Could you check a few things on this model? Use its own coordinates, in mm. Face numbers are marked on the shaded views. A direction names the side the tool comes from. Round coordinates to 2 decimals unless told otherwise and drop trailing zeros. Loops run counter-clockwise (first coordinate to the right, second up) from the corner with the lowest first, then second, coordinate; pieces in that order, holes last. Notation, with made-up numbers: (17.5, 63.25) -> (60.5, 63.25) arc R14 cw to (60.5, 83.25) -> close; hole circle Ø10 at (10, -35.75). An arc over 180 degrees is marked (long way). Put each result on its own line as item: value. Start each with the question number.
1. Imagine slicing it at A-A, the plane x = 0. Please give me the cut outline in (y, z), and give its area (3 significant figures).
2. Which directions (+Z, -Z, +X, -X, +Y, -Y) give clear straight access to the entire face, cutting with the end or side of a thin tool? Please do the marked faces 1, 2 and 3.
3. Imagine slicing it at B-B, the plane y = 8. Please give me the cut outline in (x, z).
4. I'm going to push flat-ended pins straight in: P1, Ø7, axis at x = 16, y = 12, coming from the +Z side; P2, Ø5, axis at y = 12, z = 8.5, coming from the +X side; P3, Ø1.2, axis at y = 10.5, z = 8.5, coming from the +X side. Where does each tip first touch, or does it pass through?
5. Imagine slicing it at D-D, the plane x = 14. Please give me the cut outline in (y, z).
6. If we mould it in two halves opening along Z, with no side actions, what happens to the marked faces 4, 5 and 6? For each: pulls with the +Z half, pulls with the -Z half, needs draft (parallel to the pull), parting line crosses it, or undercut.
7. I need wall thicknesses on line 1 (X direction, y = 2.65, z = -8); line 2 (X direction, y = 7.5, z = 10); line 3 (Y direction, x = 2.5, z = -10.75). Which ranges of each line are inside material? Lowest first, please. Write a range as [from, to].
8. Imagine slicing it at C-C, the plane y = 4.5. Please give me the cut outline in (x, z).
```python
from build123d import *

# Parameters (mm, degrees)
SKETCH1_R           = 1.05
BOSS_EXTRUDE1_DEPTH = 6
SKETCH2_W           = 14
SKETCH2_H           = 25
SKETCH2_W_2         = 6
SKETCH2_H_2         = 22
BOSS_EXTRUDE2_DEPTH = 10
FILLET1_R           = 1
CUT_EXTRUDE2_START  = -6
CUT_EXTRUDE2_DEPTH  = 6
FILLET2_R           = 2
CUT_EXTRUDE3_DEPTH  = 2
CUT_EXTRUDE4_REACH  = 36.587
SKETCH9_R           = 1
BOSS_EXTRUDE3_DEPTH = 1
FILLET3_R           = 1
SKETCH13_R          = 2
CUT_EXTRUDE5_DEPTH  = 2
CUT_EXTRUDE6_DEPTH  = 10
SKETCH15_R          = 1
CUT_EXTRUDE7_DEPTH  = 32.436443819
FILLET4_R           = 5


with BuildPart() as part:
    # Sketch1 → Boss-Extrude1 (new body)
    with BuildSketch(Plane(origin=(0, 0, 0), x_dir=(1, 0, 0), z_dir=(0, 1, 0))):
        Polygon((19, -4.5), (19, 5), (19, 12.5), (-19, 12.5), (-19, 5), (-19, -4.5), (-19, -5), (-19, -12.5), (19, -12.5), (19, -5), align=None)
        with Locations(Location((16, -8, 0), (0, 0, 270))):
            Circle(SKETCH1_R, mode=Mode.SUBTRACT)
        with Locations(Location((0, -8, 0), (0, 0, 270))):
            Circle(SKETCH1_R, mode=Mode.SUBTRACT)
        with Locations(Location((16, 8, 0), (0, 0, 270))):
            Circle(SKETCH1_R, mode=Mode.SUBTRACT)
        with Locations(Location((0, 8, 0), (0, 0, 270))):
            Circle(SKETCH1_R, mode=Mode.SUBTRACT)
        with Locations(Location((-16, -8, 0), (0, 0, 270))):
            Circle(SKETCH1_R, mode=Mode.SUBTRACT)
        with Locations(Location((-16, 8, 0), (0, 0, 270))):
            Circle(SKETCH1_R, mode=Mode.SUBTRACT)
    extrude(amount=BOSS_EXTRUDE1_DEPTH)

    # Sketch2 → Boss-Extrude2 (add)
    with BuildSketch(Plane(origin=(0, 6, 0), x_dir=(1, 0, 0), z_dir=(0, 1, 0))):
        with Locations((-12, 0)):
            Rectangle(SKETCH2_W, SKETCH2_H)
        with Locations((8, 0)):
            Rectangle(SKETCH2_W_2, SKETCH2_H_2)
    extrude(amount=BOSS_EXTRUDE2_DEPTH)

    # Fillet1
    fillet1_edges = [part.edges().sort_by_distance(p)[0] for p in [
        (8, 6, -11),
        (8, 6, 11),
    ]]
    fillet(fillet1_edges, radius=FILLET1_R)

    # Sketch7 → Cut-Extrude2 (cut)
    with BuildSketch(Plane(origin=(11, 0, 0), x_dir=(0, 0, -1), z_dir=(1, 0, 0)).offset(CUT_EXTRUDE2_START)):
        Polygon((-11, 11), (-9, 16), (9, 16), (11, 11), (15.487403983, 11), (15.487403983, 19.998448993), (-12.222391387, 19.998448993), (-12.222391387, 11), align=None)
    extrude(amount=CUT_EXTRUDE2_DEPTH, mode=Mode.SUBTRACT)

    # Fillet2
    fillet2_edges = [part.edges().sort_by_distance(p)[0] for p in [
        (8, 11, 11),
        (8, 16, 9),
        (8, 16, -9),
        (8, 11, -11),
    ]]
    fillet(fillet2_edges, radius=FILLET2_R)

    # Sketch8 → Cut-Extrude3 (cut)
    with BuildSketch(Plane(origin=(11, 0, 0), x_dir=(0, 0, -1), z_dir=(1, 0, 0))):
        Polygon((-5.690598923, 11), (-6.845299462, 13), (-9.154700538, 13), (-10.309401077, 11), (-9.154700538, 9), (-6.845299462, 9), align=None)
    cut_extrude3 = extrude(amount=-CUT_EXTRUDE3_DEPTH, mode=Mode.SUBTRACT)

    # Sketch9 → Cut-Extrude4 (cut, up to next)
    with BuildSketch(Plane(origin=(9, 0, 0), x_dir=(0, 0, -1), z_dir=(1, 0, 0)), mode=Mode.PRIVATE) as cut_extrude4_sk1:
        with Locations((-8, 11)):
            Circle(SKETCH9_R)
    cut_extrude4_tool1 = extrude(cut_extrude4_sk1.sketch, amount=-CUT_EXTRUDE4_REACH, mode=Mode.PRIVATE) & part.part
    cut_extrude4 = cut_extrude4_tool1.solids().sort_by_distance((9, 11, 8))[0]
    add(cut_extrude4, mode=Mode.SUBTRACT)

    # Mirror1: Cut-Extrude3, Cut-Extrude4 across plane
    add(cut_extrude3.mirror(Plane.XY), mode=Mode.SUBTRACT)
    add(cut_extrude4.mirror(Plane.XY), mode=Mode.SUBTRACT)

    # Sketch11 → Boss-Extrude3 (add, symmetric)
    with BuildSketch(Plane.XY):
        Polygon((19, 6), (11, 16), (11, 6), align=None)
    extrude(amount=BOSS_EXTRUDE3_DEPTH, both=True)

    # Fillet3
    # the kernel refuses this fillet: 1 mm, written as the material it adds along each edge
    with BuildSketch(Plane(origin=(8.5, 6, 1), x_dir=(0, 1, 0), z_dir=(1, 0, 0))) as fillet3_piece_1_section:
        with BuildLine():
            CenterArc((FILLET3_R, FILLET3_R), FILLET3_R, 180, 90)
            Line((0, FILLET3_R), (0, 0))
            Line((0, 0), (FILLET3_R, 0))
        make_face()
    fillet3_piece_1 = extrude(amount=10.5, mode=Mode.PRIVATE)
    fillet3_piece_1 = split(fillet3_piece_1, bisect_by=Plane(origin=(15.279807261, 10.650240923, 1.226395114), z_dir=(-0.7808688094430304, -0.6246950475544243, 0)), keep=Keep.TOP, mode=Mode.PRIVATE)
    add(fillet3_piece_1)
    with BuildSketch(Plane(origin=(11, 16, 1), x_dir=(0, 0, 1), z_dir=(0, -1, 0))) as fillet3_piece_2_section:
        with BuildLine():
            CenterArc((FILLET3_R, -FILLET3_R), FILLET3_R, 90, 90)
            Line((0, -FILLET3_R), (0, 0))
            Line((0, 0), (FILLET3_R, 0))
        make_face()
    fillet3_piece_2 = extrude(amount=12.5, mode=Mode.PRIVATE)
    fillet3_piece_2 = split(fillet3_piece_2, bisect_by=Plane(origin=(13.592508379, 12.759364526, 1.22990039), z_dir=(-0.7808688094430304, -0.6246950475544243, 0)), keep=Keep.TOP, mode=Mode.PRIVATE)
    add(fillet3_piece_2)
    with BuildSketch(Plane(origin=(8.5, 6, -1), x_dir=(0, 0, -1), z_dir=(1, 0, 0))) as fillet3_piece_3_section:
        with BuildLine():
            CenterArc((FILLET3_R, FILLET3_R), FILLET3_R, 180, 90)
            Line((0, FILLET3_R), (0, 0))
            Line((0, 0), (FILLET3_R, 0))
        make_face()
    fillet3_piece_3 = extrude(amount=10.5, mode=Mode.PRIVATE)
    fillet3_piece_3 = split(fillet3_piece_3, bisect_by=Plane(origin=(15.279807261, 10.650240923, -1.226395114), z_dir=(-0.7808688094430304, -0.6246950475544243, 0)), keep=Keep.TOP, mode=Mode.PRIVATE)
    add(fillet3_piece_3)
    with BuildSketch(Plane(origin=(11, 16, -1), x_dir=(0, 0, -1), z_dir=(0, -1, 0))) as fillet3_piece_4_section:
        with BuildLine():
            CenterArc((FILLET3_R, FILLET3_R), FILLET3_R, 180, 90)
            Line((0, FILLET3_R), (0, 0))
            Line((0, 0), (FILLET3_R, 0))
        make_face()
    fillet3_piece_4 = extrude(amount=12.5, mode=Mode.PRIVATE)
    fillet3_piece_4 = split(fillet3_piece_4, bisect_by=Plane(origin=(13.592508379, 12.759364526, -1.22990039), z_dir=(-0.7808688094430304, -0.6246950475544243, 0)), keep=Keep.TOP, mode=Mode.PRIVATE)
    add(fillet3_piece_4)

    # Sketch13 → Cut-Extrude5 (cut)
    with BuildSketch(Plane(origin=(0, 6, 0), x_dir=(1, 0, 0), z_dir=(0, 1, 0))):
        with Locations(Location((0, -8, 0), (0, 0, 270))):
            Circle(SKETCH13_R)
        with Locations(Location((0, 8, 0), (0, 0, 270))):
            Circle(SKETCH13_R)
    extrude(amount=-CUT_EXTRUDE5_DEPTH, mode=Mode.SUBTRACT)

    # Sketch14 → Cut-Extrude6 (cut)
    with BuildSketch(Plane.ZY.offset(19)):
        with BuildLine():
            Line((-4.987800212, 11.218644984), (-4.987800212, 6))
            Line((-4.987800212, 6), (-16.528108282, 6))
            Line((-16.528108282, 6), (-16.528108282, 44.040536724))
            Line((-16.528108282, 44.040536724), (16.528108282, 44.040536724))
            Line((16.528108282, 44.040536724), (16.528108282, 6))
            Line((16.528108282, 6), (4.987800212, 6))
            Line((4.987800212, 6), (4.987800212, 11.218644984))
            ThreePointArc((4.987800212, 11.218644984), (0, 10.3), (-4.987800212, 11.218644984))
        make_face()
    extrude(amount=-CUT_EXTRUDE6_DEPTH, mode=Mode.SUBTRACT)

    # Sketch15 → Cut-Extrude7 (cut, through all)
    with BuildSketch(Plane(origin=(-5, 0, 0), x_dir=(0, 0, -1), z_dir=(1, 0, 0))):
        with Locations((-8, 11)):
            Circle(SKETCH15_R)
        with Locations((8, 11)):
            Circle(SKETCH15_R)
    extrude(amount=-CUT_EXTRUDE7_DEPTH, mode=Mode.SUBTRACT)

    # Fillet4
    # the kernel refuses this fillet: 5 mm, written as the material it adds along each edge
    with BuildSketch(Plane(origin=(-9, 24.3, 0), x_dir=(0, -0.30847325638563394, 0.9512330156669516), z_dir=(0, 0.9512330156669516, 0.30847325638563394))) as fillet4_piece_1_section:
        with BuildLine():
            CenterArc((14 - FILLET4_R, -FILLET4_R), FILLET4_R, 0, 90)
            Line((14, -FILLET4_R), (14, 0))
            Line((14, 0), (14 - FILLET4_R, 0))
        make_face()
    fillet4_piece_1 = revolve(axis=Axis((-9, 24.3, 0), (1, 0, 0)), revolution_arc=144.065508201, mode=Mode.PRIVATE)
    fillet4_piece_1 = split(fillet4_piece_1, bisect_by=Plane(origin=(-10.130683899, 16, -3.44e-07), z_dir=(0, -1, 0)), keep=Keep.TOP, mode=Mode.PRIVATE)
    fillet4_piece_1 = split(fillet4_piece_1, bisect_by=Plane(origin=(-10.130683899, 11.770838436, 4.987800212), z_dir=(0, 0, -1)), keep=Keep.TOP, mode=Mode.PRIVATE)
    fillet4_piece_1 = split(fillet4_piece_1, bisect_by=Plane(origin=(-10.130683899, 11.770838436, -4.987800212), z_dir=(0, 0, 1)), keep=Keep.TOP, mode=Mode.PRIVATE)
    add(fillet4_piece_1)


solid = part.part
```
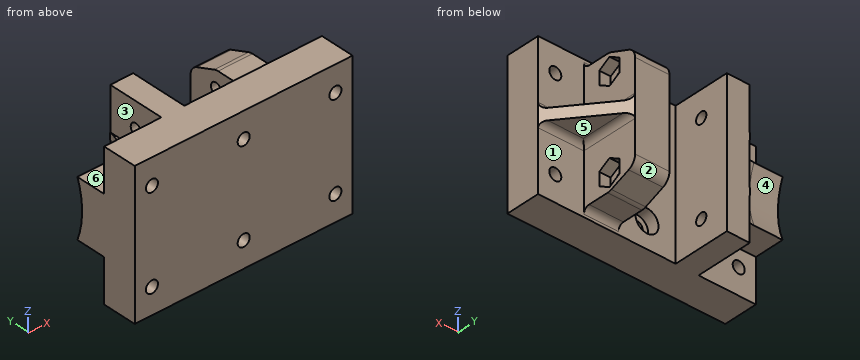
Entries:
1. outline: (0, -12.5) -> (6, -12.5) -> (6, -10) -> (4, -10) -> (4, -9.05) -> (0, -9.05) -> close; (0, -6.95) -> (4, -6.95) -> (4, -6) -> (6, -6) -> (6, 6) -> (4, 6) -> (4, 6.95) -> (0, 6.95) -> close; (0, 9.05) -> (4, 9.05) -> (4, 10) -> (6, 10) -> (6, 12.5) -> (0, 12.5) -> close
1. area: 117 mm^2
2. face 1: +Y
2. face 2: -Z, +X, +Y
2. face 3: +Z, -X, +Y
3. outline: (-19, -4.99) -> (-9, -4.99) -> (-9, -12.5) -> (-5, -12.5) -> (-5, 12.5) -> (-9, 12.5) -> (-9, 4.99) -> (-19, 4.99) -> close; (5, -11) -> (11, -11) -> (11, -2) arc R1 cw to (12, -1) -> (17.4, -1) -> (17.4, 1) -> (12, 1) arc R1 cw to (11, 2) -> (11, 11) -> (5, 11) -> close
4. P1: z = 1
4. P2: x = 11
4. P3: x = 9
5. outline: (0, -12.5) -> (6, -12.5) -> (6, -2) arc R1 cw to (7, -1) -> (12.25, -1) -> (12.25, 1) -> (7, 1) arc R1 cw to (6, 2) -> (6, 12.5) -> (0, 12.5) -> close
6. face 4: undercut
6. face 5: pulls with the -Z half
6. face 6: pulls with the +Z half
7. line 1: [-19, -17.05], [-14.95, -1.05], [1.05, 14.95], [17.05, 19]
7. line 2: [-9, -5], [5, 11]
7. line 3: [0, 6]
8. outline: (-19, -12.5) -> (19, -12.5) -> (19, 12.5) -> (-19, 12.5) -> close; hole circle Ø2.1 at (-16, -8); hole circle Ø2.1 at (-16, 8); hole circle Ø4 at (0, -8); hole circle Ø4 at (0, 8); hole circle Ø2.1 at (16, -8); hole circle Ø2.1 at (16, 8)
